Check sheet for the modelled part. Datum: model origin and axes. Units: mm. A direction names the side the tool comes from. Give positions to 0.01 mm unless a question says otherwise; leave off trailing zeros. Write each loop counter-clockwise with the first axis right and the second up, starting at its lowest first coordinate (ties: lowest second). Pieces come first, ordered by that corner, then holes. Notation, with made-up numbers: M -12,-1.75 L 37,-1.75 A8 cw 37,10.25 Z; hole C 24.5,10 d2. An arc over 180 degrees is marked long. Use CSV: the item, a comma, the result in double quotes. Start each with the question number.
1. Cross-section at D-D, the plane x = 0. Enter the section's corners in (y, z).
2. Mould release check, pull along Y, two halves, no side actions. Record for faces 1 (the face through (4, -1, 0)), 2 (the face through (5.93, 7.73, -0.02)), 3 (the face through (2.5, 7.1, 0)): +Y half, -Y half, draft (parallel to the pull), parting line (faces both ways), or undercut.
3. Depth check by flat-ended pin: P1, Ø2, axis at x = 3.9, z = 0, coming from the -Y side (3 decimals); P2, Ø1.6, axis at y = 0.5, z = 0.5, coming from the +X side; P3, Ø4, axis at x = 2.5, y = -0.5, coming from the -Z side; P4, Ø4, axis at x = -3, z = 1, coming from the +Y side. Enter the tip coordinate at first touch or a pass-through.
4. Cross-section at B-B, the plane x = -3.9. Enter the section's corners in (y, z).
5. Cross-section at C-C, the plane y = 7.5. Enter the section's corners in (x, z).
6. Access from +Z, -Z, +X, -X, +Y, -Y to the whole of each face (thin tool, end or side, straight path). Record for faces 4 (the face through (-4, -1, 0)), 5 (the face through (2.48, 7.07, 1.4)), 6 (the face through (5, 7, 0)).
7. Scan lines: line 1 (Z direction, x = -3.9, y = 7.95); line 2 (X direction, y = 8.4, z = 0); line 3 (X direction, y = 7.7, z = 0). Record each from-to range of solid material in increasing order.
8. Cross-section at A-A, the plane y = 5.5. Enter the section's corners in (x, z).
from build123d import *

# Parameters (mm, degrees)
BOSS_EXTRUDE1_DEPTH     = 7.05
SKETCH4_R               = 3.5
BOSS_EXTRUDE2_DEPTH     = 0.75
SKETCH5_R               = 1.125
BOSS_EXTRUDE3_DEPTH     = 2.4
SKETCH6_R               = 1
BOSS_EXTRUDE4_DEPTH     = 1.2
SKETCH7_R               = 1.125
BOSS_EXTRUDE5_DEPTH     = 2.4
SKETCH8_R               = 1
BOSS_EXTRUDE6_DEPTH     = 1.2
BOSS_EXTRUDE8_DEPTH     = 4.8
CUT_EXTRUDE1_DEPTH      = 4.8
CUT_EXTRUDE2_DEPTH      = 4.9
CUT_EXTRUDE2_DEPTH_BACK = 4.9


with BuildPart() as part:
    # Sketch2 → Boss-Extrude1 (new body, symmetric)
    with BuildSketch(Plane(origin=(0, 0, 0), x_dir=(0, 0, -1), z_dir=(1, 0, 0))):
        with BuildLine():
            ThreePointArc((-2.343074903, 2.6), (0, 3.5), (2.343074903, 2.6))
            Line((2.343074903, 2.6), (3.9, 2.6))
            Line((3.9, 2.6), (3.9, 4.7))
            Line((3.9, 4.7), (-3.9, 4.7))
            Line((-3.9, 4.7), (-3.9, 2.6))
            Line((-3.9, 2.6), (-2.343074903, 2.6))
        make_face()
    extrude(amount=BOSS_EXTRUDE1_DEPTH, both=True)

    # Sketch4 → Boss-Extrude2 (add, symmetric)
    with BuildSketch(Plane(origin=(0, 0, 0), x_dir=(0, 0, -1), z_dir=(1, 0, 0))):
        Circle(SKETCH4_R)
    extrude(amount=BOSS_EXTRUDE2_DEPTH, both=True)

    # Sketch5 → Boss-Extrude3 (add)
    with BuildSketch(Plane(origin=(0.75, 0, 0), x_dir=(0, 0, -1), z_dir=(1, 0, 0))):
        Circle(SKETCH5_R)
    extrude(amount=BOSS_EXTRUDE3_DEPTH)

    # Sketch6 → Boss-Extrude4 (add)
    with BuildSketch(Plane(origin=(3.15, 0, 0), x_dir=(0, 0, -1), z_dir=(1, 0, 0))):
        Circle(SKETCH6_R)
    extrude(amount=BOSS_EXTRUDE4_DEPTH)

    # Sketch7 → Boss-Extrude5 (add)
    with BuildSketch(Plane.ZY.offset(0.75)):
        Circle(SKETCH7_R)
    extrude(amount=BOSS_EXTRUDE5_DEPTH)

    # Sketch8 → Boss-Extrude6 (add)
    with BuildSketch(Plane.ZY.offset(3.15)):
        Circle(SKETCH8_R)
    extrude(amount=BOSS_EXTRUDE6_DEPTH)

    # Sketch9 → Boss-Extrude8 (add)
    with BuildSketch(Plane(origin=(0, 4.7, 0), x_dir=(1, 0, 0), z_dir=(0, 1, 0))):
        with BuildLine():
            Line((2.9, -2.4), (4.9, -2.4))
            ThreePointArc((4.9, -2.4), (5.310050506, -1.410050506), (6.3, -1))
            Line((6.3, -1), (6.3, 1))
            ThreePointArc((6.3, 1), (5.310050506, 1.410050506), (4.9, 2.4))
            Line((4.9, 2.4), (2.9, 2.4))
            ThreePointArc((2.9, 2.4), (2.489949494, 1.410050506), (1.5, 1))
            Line((1.5, 1), (1.5, -1))
            ThreePointArc((1.5, -1), (2.489949494, -1.410050506), (2.9, -2.4))
        make_face()
        with BuildLine():
            Line((-6.3, -1), (-6.3, 1))
            ThreePointArc((-6.3, 1), (-5.310050506, 1.410050506), (-4.9, 2.4))
            Line((-4.9, 2.4), (-2.9, 2.4))
            ThreePointArc((-2.9, 2.4), (-2.489949494, 1.410050506), (-1.5, 1))
            Line((-1.5, 1), (-1.5, -1))
            ThreePointArc((-1.5, -1), (-2.489949494, -1.410050506), (-2.9, -2.4))
            Line((-2.9, -2.4), (-4.9, -2.4))
            ThreePointArc((-4.9, -2.4), (-5.310050506, -1.410050506), (-6.3, -1))
        make_face()
    extrude(amount=BOSS_EXTRUDE8_DEPTH)

    # Sketch10 → Cut-Extrude1 (cut)
    with BuildSketch(Plane(origin=(0, 9.5, 0), x_dir=(1, 0, 0), z_dir=(0, 1, 0))):
        with BuildLine():
            Line((5, 0.866025404), (5, -0.866025404))
            ThreePointArc((5, -0.866025404), (2.5, 0), (5, 0.866025404))
        make_face()
        with BuildLine():
            Line((-5, 0.866025404), (-5, -0.866025404))
            ThreePointArc((-5, -0.866025404), (-2.5, 0), (-5, 0.866025404))
        make_face()
    extrude(amount=-CUT_EXTRUDE1_DEPTH, mode=Mode.SUBTRACT)

    # Sketch12 → Cut-Extrude2 (cut, two sides)
    with BuildSketch(Plane.XY) as cut_extrude2_sk:
        Polygon((5.55, 9.5), (6.3, 9.5), (6.3, 6), align=None)
        Polygon((-6.3, 6), (-5.55, 9.5), (-6.3, 9.5), align=None)
    extrude(amount=CUT_EXTRUDE2_DEPTH, mode=Mode.SUBTRACT)
    extrude(cut_extrude2_sk.sketch, amount=-CUT_EXTRUDE2_DEPTH_BACK, mode=Mode.SUBTRACT)


solid = part.part
Worked answers:
1,outline,"M 2.6,-3.9 L 4.7,-3.9 L 4.7,3.9 L 2.6,3.9 L 2.6,2.34 A3.5 ccw long 2.6,-2.34 Z"
2,face 1,"undercut"
2,face 2,"+Y half"
2,face 3,"draft"
3,P1,"stops at y = -1.125"
3,P2,"stops at x = 4.35"
3,P3,"stops at z = -3.5"
3,P4,"stops at y = 9.5"
4,outline,"C 0,0 d2; M 2.6,-3.9 L 4.7,-3.9 L 4.7,-2.4 L 9.5,-2.4 L 9.5,-1.4 L 4.7,-1.4 L 4.7,1.4 L 9.5,1.4 L 9.5,2.4 L 4.7,2.4 L 4.7,3.9 L 2.6,3.9 L 2.6,2.34 A3.5 cw 2.6,-2.34 Z"
5,outline,"M -5.98,-1.04 A1.4 cw -4.9,-2.4 L -2.9,-2.4 A1.4 cw -1.5,-1 L -1.5,1 A1.4 cw -2.9,2.4 L -4.9,2.4 A1.4 cw -5.98,1.04 Z; M 1.5,-1 A1.4 cw 2.9,-2.4 L 4.9,-2.4 A1.4 cw 5.98,-1.04 L 5.98,1.04 A1.4 cw 4.9,2.4 L 2.9,2.4 A1.4 cw 1.5,1 Z; hole M -5,-0.87 A1.4 ccw long -5,0.87 Z; hole M 5,-0.87 L 5,0.87 A1.4 ccw long Z"
6,face 4,"-X"
6,face 5,"+Z, +Y"
6,face 6,"+Y"
7,line 1,"z = -2.4 to -1.4, 1.4 to 2.4"
7,line 2,"x = -5.79 to -5, -2.5 to -1.5, 1.5 to 2.5, 5 to 5.79"
7,line 3,"x = -5.94 to -5, -2.5 to -1.5, 1.5 to 2.5, 5 to 5.94"
8,outline,"M -6.3,-1 A1.4 cw -4.9,-2.4 L -2.9,-2.4 A1.4 cw -1.5,-1 L -1.5,1 A1.4 cw -2.9,2.4 L -4.9,2.4 A1.4 cw -6.3,1 Z; M 1.5,-1 A1.4 cw 2.9,-2.4 L 4.9,-2.4 A1.4 cw 6.3,-1 L 6.3,1 A1.4 cw 4.9,2.4 L 2.9,2.4 A1.4 cw 1.5,1 Z; hole M -5,-0.87 A1.4 ccw long -5,0.87 Z; hole M 5,-0.87 L 5,0.87 A1.4 ccw long Z"
